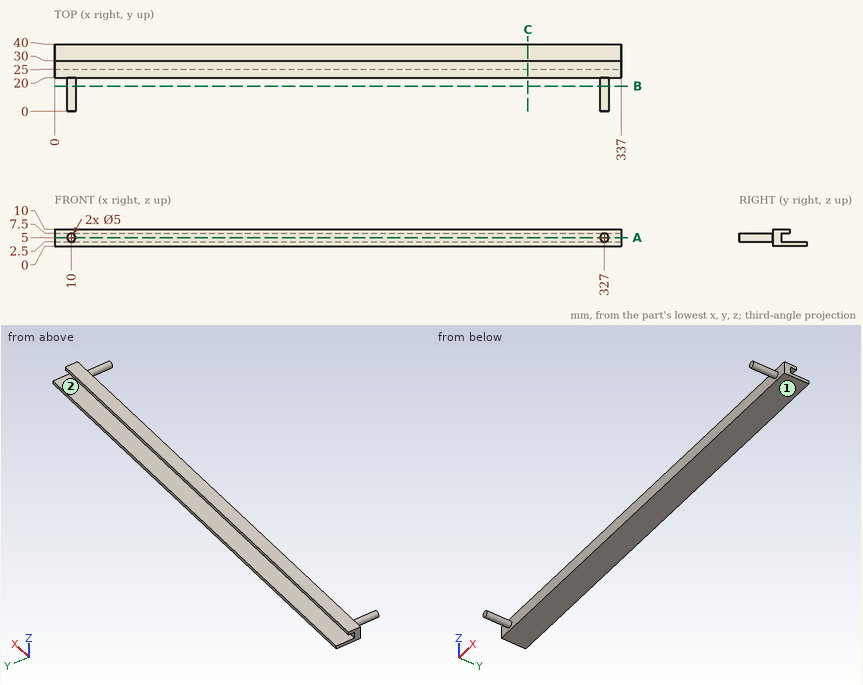
Could you check a few things on this drawing? It's one solid part, dimensions in mm from its lowest x, y, z. A direction names the side the tool comes from. Give positions to 0.01 mm unless a question says otherwise; leave off trailing zeros. Order: outer loops, then holes, each group sorted by start corner. A loop starts at its lowest first (then second) coordinate and runs counter-clockwise, first axis right, second up. Notation, with made-up numbers: M 64.25,-11.5 L 112.25,-11.5 A15 ccw 112.25,8.5 Z; hole C 4,89 d3. An arc over 180 degrees is marked long. Use one line per item in the form item = value. Start each with the question number.
Item 1: Will these pins go through, and if not, where does the flat tip stop? pin 1 Ø4 at (x, z) = (52.5, 8.5) entering from +Y; pin 2 Ø6 at (x, z) = (42, 3) entering from -Y; pin 3 Ø1.5 at (x, y) = (174.5, 26.5) entering from -Z; pin 4 Ø4 at (x, z) = (112.5, 5) entering from +Y.
Item 2: If I drill on line 1 along Y through (x, z) = (22, 3.5); line 2 along Z through (x, y) = (249, 30.5); line 3 along Z through (x, y) = (51.5, 27), over which ranges is the centre line in solid material (lowest first)?
Item 3: If we section it at C-C (x = 281.5): Write out the boundary of the cut face in (y, z), then the cut area to 3 significant figures.
Item 4: If we section it at A-A (z = 5): Write out the boundary of the cut face in (x, y), then the cut area to 4 significant figures.
Item 5: For the marked faces 1 and 2, which set-ups out of +Z, -Z, +X, -X, +Y, -Y let a thin tool reach every point of the face, with its end or its side?
Item 6: If we section it at B-B (y = 15): Write out the boundary of the cut face in (x, z).
Outcome:
q1.pin_1 = 30
q1.pin_2 = 20
q1.pin_3 = 0
q1.pin_4 = 25
q2.line_1 = 20 to 25
q2.line_2 = 0 to 2.5
q2.line_3 = 0 to 2.5, 7.5 to 10
q3.outline = M 20,0 L 40,0 L 40,2.5 L 25,2.5 L 25,7.5 L 30,7.5 L 30,10 L 20,10 Z
q3.area = 100 mm2
q4.outline = M 0,20 L 7.5,20 L 7.5,0 L 12.5,0 L 12.5,20 L 324.5,20 L 324.5,0 L 329.5,0 L 329.5,20 L 337,20 L 337,25 L 0,25 Z
q4.area = 1,885 mm2
q5.face_1 = -Z, +X, -X, +Y, -Y
q5.face_2 = +X, -X, +Y
q6.outline = C 10,5 d5; C 327,5 d5
